Check sheet for the modelled part. Datum: model origin and axes. Units: mm. A direction names the side the tool comes from. Give positions to 0.01 mm unless a question says otherwise; leave off trailing zeros. Order: outer loops, then holes, each group sorted by start corner. A loop starts at its lowest first (then second) coordinate and runs counter-clockwise, first axis right, second up.
```python
from build123d import *

# Parameters (mm, degrees)
BOX017_W          = 14
BOX017_H          = 14
BOX017_DEPTH      = 4.5
CYLINDER095_R     = 2
CYLINDER095_DEPTH = 8
PAD089_DEPTH      = 1
SKETCH155_W       = 14.5
SKETCH155_H       = 14.5
SKETCH156_W       = 11
SKETCH156_H       = 11
PAD090_DEPTH      = 9
SKETCH158_W       = 7.5
SKETCH158_H       = 6
PAD092_DEPTH      = 1


with BuildPart() as part:
    # Box017 → Box017 (join)
    with BuildSketch(Plane(origin=(7, -7, 0), x_dir=(-1, 0, 0), z_dir=(0, 0, -1))):
        with Locations((7, 7)):
            Rectangle(BOX017_W, BOX017_H)
    extrude(amount=BOX017_DEPTH)

    # Cylinder095 → Cylinder095 (join)
    with BuildSketch(Plane(origin=(0, 0, 0), x_dir=(-1, 0, 0), z_dir=(0, 0, -1))):
        Circle(CYLINDER095_R)
    extrude(amount=CYLINDER095_DEPTH)

    # Sketch154 → Pad089 (join)
    with BuildSketch(Plane.XY):
        Polygon((-7.75, 5.75), (-7.75, 7.75), (-2.75, 7.75), (-2.75, 7), (2.75, 7), (2.75, 7.75), (7.75, 7.75), (7.75, 5.75), (7, 5.75), (7, -5.75), (7.75, -5.75), (7.75, -7.75), (2.75, -7.75), (2.75, -7), (-2.75, -7), (-2.75, -7.75), (-7.75, -7.75), (-7.75, -5.75), (-7, -5.75), (-7, 5.75), align=None)
    extrude(amount=PAD089_DEPTH)

    # Sketch155 → AdditiveLoft002 section 0
    with BuildSketch(Plane.XY):
        Rectangle(SKETCH155_W, SKETCH155_H)
    # Sketch156 → AdditiveLoft002 section 1
    with BuildSketch(Plane.XY.offset(6)):
        Rectangle(SKETCH156_W, SKETCH156_H)
    loft()

    # Sketch157 → Pad090 (join)
    with BuildSketch(Plane.XY):
        Polygon((-0.6, 1.907878), (0.6, 1.907878), (0.6, 0.6), (1.907878, 0.6), (1.907878, -0.6), (0.6, -0.6), (0.6, -1.907878), (-0.6, -1.907878), (-0.6, -0.6), (-1.907878, -0.6), (-1.907878, 0.6), (-0.6, 0.6), align=None)
    extrude(amount=PAD090_DEPTH)

    # Sketch158 → Pad092 (join)
    with BuildSketch(Plane.XY.offset(5)):
        Rectangle(SKETCH158_W, SKETCH158_H)
    extrude(amount=PAD092_DEPTH)


with BuildPart() as part_1:
    # Body181003 placement: moved
    add(part.part.moved(Location((0, 8, 0))))


solid = part_1.part
```
(1) Cross-section at A-A on z = 7.25. Enter the section's corners in (x, y), then the cut area to 3 significant figures.
Response values:
outline: (-1.91, 7.4) - (-0.6, 7.4) - (-0.6, 6.09) - (0.6, 6.09) - (0.6, 7.4) - (1.91, 7.4) - (1.91, 8.6) - (0.6, 8.6) - (0.6, 9.91) - (-0.6, 9.91) - (-0.6, 8.6) - (-1.91, 8.6) - close
area: 7.72 mm2
(2) Cross-section at B-B on z = -1.75. Enter the section's corners in (x, y).
Response values:
outline: (-7, 1) - (7, 1) - (7, 15) - (-7, 15) - close
(3) Set-up check for faces 1 (the face through (-7, 8, -2)), 2 (the face through (1, 7.4, 7)), 3 (the face through (-1, 8.6, 7)), 4 (the face through (-1.908, 8, 7)): record each of +Z, -Z, +X, -X, +Y, -Y from which the full face is reachable in a straight line by a thin tool's end or side.
Response values:
face 1: -Z, -X, +Y, -Y
face 2: +Z, +X, -Y
face 3: +Z, -X, +Y
face 4: +Z, -X, +Y, -Y
(4) Material ranges on L1, parallel to X at y = 2, z = -2.5; L2, parallel to Z at x = 2.5, y = 10; L3, parallel to Y at x = 1, z = -3.25, recorded low to high.
Response values:
L1: x = -7 to 7
L2: z = -4.5 to 6
L3: y = 1 to 15
(5) Gauge pin test, flat ends, axial feed: pin 1 Ø3 at (x, y) = (2.5, 11) entering from -Z; pin 2 Ø1 at (y, z) = (8, 7) entering from +X; pin 3 Ø5 at (y, z) = (9, -4.5) entering from -X. Record the tip position at first contact, or that the pin passes through.
Response values:
pin 1: stops at z = -4.5
pin 2: stops at x = 1.91
pin 3: stops at x = -7
(6) Cross-section at C-C on z = -5.5. Enter the section's corners in (x, y).
Response values:
outline: circle Ø4 at (0, 8)
